Geometry: see drawing. Coordinates: mm, zero at the bounding-box minimum. Coordinates: 2 decimals unless noted, no trailing zeros. Order: outer loops, then holes, each group sorted by start corner. A loop starts at its lowest first (then second) coordinate and runs counter-clockwise, first axis right, second up.
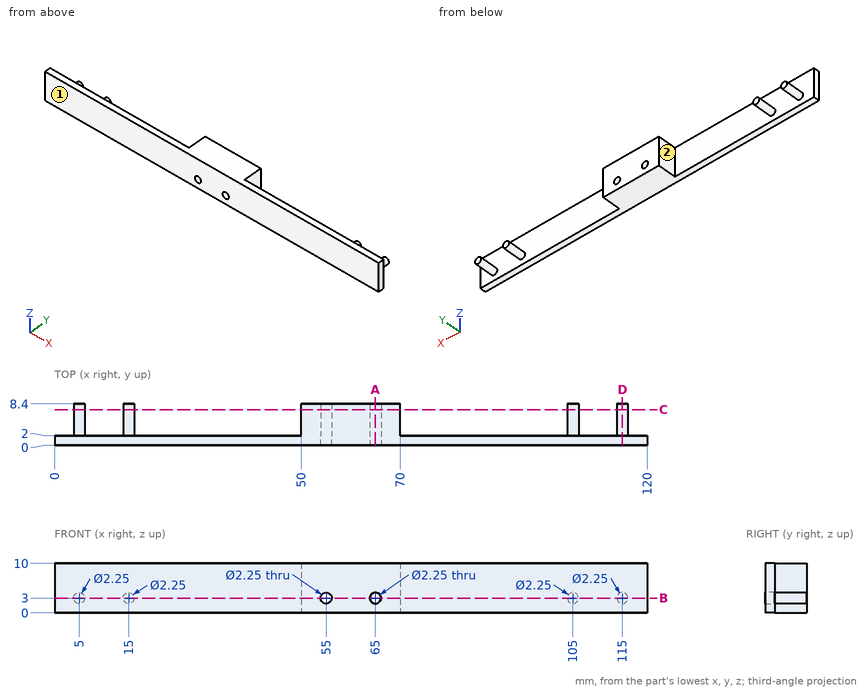
Q1. Pin query (flat end, axial travel): P1, Ø3, axis at x = 19, z = 3.5, coming from the +Y side; P2, Ø2.5, axis at x = 55, z = 3, coming from the +Y side. Return the tip coordinate at first contact, or that it passes through.
Solutions:
P1: stops at y = 2
P2: stops at y = 8.4
Q2. Section query B-B on z = 3. Give the number of separate pieces and of enclosed holes in the cut face, plus the area to 3 significant figures.
Solutions:
separate pieces: 3
enclosed holes: 0
area: 388 mm2
Q3. Section query C-C on y = 7.25. Output: boundary loops of the cut face in (x, z) (3 decimals).
Solutions:
outline: circle Ø2.25 at (5, 3); circle Ø2.25 at (15, 3); (50, 0) - (70, 0) - (70, 10) - (50, 10) - close; circle Ø2.25 at (105, 3); circle Ø2.25 at (115, 3); hole circle Ø2.25 at (55, 3); hole circle Ø2.25 at (65, 3)
Q4. Material intervals for line 1 along X through (y, z) = (0.85, 3) (3 decimals); line 2 along Y through (x, z) = (32.5, 3); line 3 along X through (y, z) = (3.25, 6.5), sorted ascending.
Solutions:
line 1: x = 0 to 53.875, 56.125 to 63.875, 66.125 to 120
line 2: y = 0 to 2
line 3: x = 50 to 70
Q5. Pull-direction query (X, two-part tool) for the marked faces 1 and 2; classes: pulls with the +X half, pulls with the -X half, needs draft (parallel to the pull), parting line crosses it, or undercut.
Solutions:
face 1: needs draft
face 2: undercut
Q6. Section query A-A on x = 65. Output: boundary loops of the cut face in (y, z) (3 decimals).
Solutions:
outline: (0, 0) - (8.4, 0) - (8.4, 1.875) - (0, 1.875) - close; (0, 4.125) - (8.4, 4.125) - (8.4, 10) - (0, 10) - close
Q7. Section query D-D on x = 115. Output: boundary loops of the cut face in (y, z) (3 decimals), plus the area to 3 significant figures.
Solutions:
outline: (0, 0) - (2, 0) - (2, 1.875) - (8.4, 1.875) - (8.4, 4.125) - (2, 4.125) - (2, 10) - (0, 10) - close
area: 34.4 mm2
